```python
from build123d import *

# Parameters (mm, degrees)
PAD_DEPTH       = 5
SKETCH056_R     = 2.35
PAD023_DEPTH    = 5
SKETCH057_W     = 23
SKETCH057_H     = 42.3
PAD024_DEPTH    = 7.5
SKETCH058_R     = 7.5
POCKET013_DEPTH = 100
FILLET_R        = 4
FILLET002_R     = 3
FILLET003_R     = 0.5


with BuildPart() as part:
    # Sketch (on Face1 of Binder) → Pad (new body)
    with BuildSketch(Plane.XY.offset(68)):
        Polygon((-21.15, 15.8466991411), (-15.8466991411, 21.15), (15.8466991411, 21.15), (21.15, 15.8466991411), (21.15, -15.8466991411), (15.8466991411, -21.15), (-15.8466991411, -21.15), (-21.15, -15.8466991411), align=None)
    extrude(amount=PAD_DEPTH)

    # Sketch056 (on Face9 of Pad) → Pad023 (join)
    with BuildSketch(Plane(origin=(0, 0, 68), x_dir=(1, 0, 0), z_dir=(0, 0, -1))):
        with Locations((15.5, 15.5)):
            Circle(SKETCH056_R)
        with Locations((15.5, -15.5)):
            Circle(SKETCH056_R)
        with Locations((-15.5, -15.5)):
            Circle(SKETCH056_R)
        with Locations((-15.5, 15.5)):
            Circle(SKETCH056_R)
    extrude(amount=PAD023_DEPTH)

    # Sketch057 (on Face5 of Pad023) → Pad024 (join)
    with BuildSketch(Plane.XY.offset(73)):
        Rectangle(SKETCH057_W, SKETCH057_H)
    extrude(amount=PAD024_DEPTH)

    # Sketch058 (on Face20 of Pad024) → Pocket013 (cut)
    with BuildSketch(Plane.XZ.offset(21.15)):
        with Locations((0, 80.5)):
            Circle(SKETCH058_R)
    extrude(amount=-POCKET013_DEPTH, mode=Mode.SUBTRACT)

    # Fillet
    fillet_edges = [part.edges().sort_by_distance(p)[0] for p in [
        (11.5, 0, 73),
        (-11.5, 0, 73),
    ]]
    fillet(fillet_edges, radius=FILLET_R)

    # Fillet002
    fillet002_edges = [part.edges().sort_by_distance(p)[0] for p in [
        (-11.5, 0, 80.5),
        (11.5, 0, 80.5),
    ]]
    fillet(fillet002_edges, radius=FILLET002_R)

    # Fillet003
    fillet003_edges = [part.edges().sort_by_distance(p)[0] for p in [
        (21.15, 0, 73),
        (-21.15, 0, 73),
    ]]
    fillet(fillet003_edges, radius=FILLET003_R)


solid = part.part
```
Model file for the job. Use its own axes, mm. A direction names the side the tool comes from. Give positions to 0.01 mm unless a question says otherwise; leave off trailing zeros. Loops run counter-clockwise (first coordinate to the right, second up) from the corner with the lowest first, then second, coordinate; pieces in that order, holes last. Notation, with made-up numbers: M 54.25,54 L 85.25,54 A24 cw 85.25,75 Z; hole C 72.5,14.25 d10. An arc over 180 degrees is marked long. Use one line per item in the form item = value.
Item 1: Slice it at D-D on x = 19.5. List the corners of the cut face in (y, z).
Filled in:
outline = M -17.5,68 L 17.5,68 L 17.5,73 L -17.5,73 Z
Item 2: Flat gauge pins, fed straight in: pin 1 Ø10 at (y, z) = (-14, 66.5) entering from -X; pin 2 Ø5.5 at (x, y) = (19, 5.5) entering from +Z; pin 3 Ø2 at (x, y) = (-0.5, 15) entering from +Z; pin 4 Ø1 at (x, y) = (13.5, -7.5) entering from +Z. Where does each tip first touch, or does it go through?
Filled in:
pin_1 = -21.15
pin_2 = 73
pin_3 = 73.15
pin_4 = 73.88
Item 3: Drill centre lines: L1, parallel to X at y = 7, z = 76; L2, parallel to X at y = 7, z = 79; L3, parallel to Z at x = -8, y = -4. Where is each one in solid material? Low to high.
Filled in:
L1 = -11.63 to -6, 6 to 11.63
L2 = -11.1 to -7.35, 7.35 to 11.1
L3 = 68 to 80.5
Item 4: Slice it at C-C on x = 0. List the corners of the cut face in (y, z).
Filled in:
outline = M -21.15,68 L 21.15,68 L 21.15,73 L -21.15,73 Z
Item 5: Slice it at A-A on y = 8. List the corners of the cut face in (x, z), and give its area (3 significant figures).
Filled in:
outline = M -21.15,68 L 21.15,68 L 21.15,72.5 A0.5 ccw 20.65,73 L 15.5,73 A4 cw 11.5,77 L 11.5,77.5 A3 ccw 8.5,80.5 L 7.5,80.5 A7.5 cw -7.5,80.5 L -8.5,80.5 A3 ccw -11.5,77.5 L -11.5,77 A4 cw -15.5,73 L -20.65,73 A0.5 ccw -21.15,72.5 Z
area = 299 mm^2
Item 6: Two-plate mould, pull along X, no slides. Class faces 4 (the flat face through (-18, 0, 73)), 5 (the flat face through (-18.535, 18.461, 70.465)), 6 (the cylindrical face through (12.703, 0.296, 74.141)), 7 (the flat face through (0, 0, 68)): released by +X, released by -X, zero draft, split by the parting line, or undercut.
Filled in:
face_4 = zero draft
face_5 = released by -X
face_6 = released by +X
face_7 = undercut
Item 7: Which spindle directions (+Z, -Z, +X, -X, +Y, -Y) get a long thin tool onto all of the face, cutting with end or side? Do faces 1 (the flat face through (15, 15, 63)), 2 (the flat face through (18, 0, 73)), 3 (the cylindrical face through (13.635, 16.93, 65.535)). Say none if no direction does.
Filled in:
face_1 = -Z, +X, -X, +Y, -Y
face_2 = +Z, +X, +Y, -Y
face_3 = -Z
Item 8: Slice it at B-B on z = 73.5. List the corners of the cut face in (x, y).
Filled in:
outline = M -13.56,-21.15 L -2.69,-21.15 L -2.69,21.15 L -13.56,21.15 Z; M 2.69,-21.15 L 13.56,-21.15 L 13.56,21.15 L 2.69,21.15 Z
